Geometry check sheet. Reference: the model listing, model coordinates, mm. A direction names the side the tool comes from. Round coordinates to 2 decimals unless told otherwise and drop trailing zeros. Write each loop counter-clockwise with the first axis right and the second up, starting at its lowest first coordinate (ties: lowest second). Pieces come first, ordered by that corner, then holes. Notation, with made-up numbers: (63.5, 21) - (109.5, 21) arc R15 cw to (109.5, 35) - close; hole circle Ø4 at (26.25, -27). An arc over 180 degrees is marked (long way). Return JSON: item names as keys, results as strings.
Autodesk Inventor part; units mm, degrees
ref_plane "Work Plane4" through (-20, 152.4, 0) normal (-1, 0, 0) x (0, -1, 0)
ref_plane "YZ Plane" through (0, 0, 0) normal (1, 0, 0) x (0, 1, 0)
ref_plane "XZ Plane" through (0, 0, 0) normal (0, 1, 0) x (-1, 0, 0)
sketch "Sketch1" plane through (0, 0, 0) normal (0, 1, 0) x (-1, 0, 0)
  circle A0 centre (0, 0) radius 20
  circle A1 centre (0, 0) radius 18.5
  dimension "d0" = 40
  dimension "d1" = 1.5
extrude "Extrusion1" add sketch "Sketch1" along normal blind 152.4
sketch "Sketch4" plane through (0, 152.4, 0) normal (0, 1, 0) x (1, 0, 0)
  circle A0 centre (0, 0) radius 18.5
  circle A1 centre (0, 0) radius 20
  point P0 (-20, 0)
ref_plane "Work Plane4" through (-20, 152.4, 0) normal (-1, 0, 0) x (0, -1, 0)
sketch "Sketch8" plane through (-20, 152.4, 0) normal (-1, 0, 0) x (0, -1, 0)
  line L0 (0, 0) -> (0, 304.8) construction
  arc A0 (-304.8, 304.8) -> (0, 0) centre (0, 304.8) ccw
  line L1 (0, 304.8) -> (-304.8, 304.8) construction
  point P0 (152.4, 0)
  dimension "d7" = 304.8
sweep "Sweep1" add profiles "Sketch4" path "Sketch8"
sketch "Sketch9" plane through (0, 457.2, 304.8) normal (0, 0, 1) x (1, 0, 0)
  circle A0 centre (0, 0) radius 18.5
  circle A1 centre (0, 0) radius 20
  point P0 (0, -457.2)
extrude "Extrusion2" add sketch "Sketch9" along normal blind 152.4
properties part number "sweep" material "ABS Plastic"
(1) Release check for a two-part mould opening along Y. For faces 1 (the face through (-6, 0, -18)), 2 (the face through (18, 451, 457.2)), 3 (the face through (8.54, 473.61, 379.93)) record: pulls with the +Y half, pulls with the -Y half, needs draft (parallel to the pull), parting line crosses it, or undercut.
Response values:
{"face 1": "pulls with the -Y half", "face 2": "needs draft", "face 3": "undercut"}
(2) Access from +Z, -Z, +X, -X, +Y, -Y to the whole of each face (thin tool, end or side, straight path). Record for faces 4 (the face through (4.01, 75.13, 18.06)), 5 (the face through (10.752, 440.336, 379.933)).
Response values:
{"face 4": "-Y", "face 5": "+Z"}
(3) Material ranges on line 1 along X through (y, z) = (196, 2.5); line 2 along Z through (x, y) = (0, 98.5); line 3 along Y through (x, z) = (15, 435.5), recorded low to high. Write a range as [from, to].
Response values:
{"line 1": "x = [-19.99, -18.49], [18.49, 19.99]", "line 2": "z = [-20, -18.5], [18.5, 20]", "line 3": "y = [443.97, 446.37], [468.03, 470.43]"}
(4) Section check B-B, the plane z = 401.5. Enter the section's corners in (x, y), plus the area to 3 significant figures.
Response values:
{"outline": "circle Ø40 at (0, 457.2); hole circle Ø37 at (0, 457.2)", "area": "181 mm^2"}
(5) Gauge pin test, flat ends, axial feed: pin 1 (12 mm diameter, centred on y = 406.5, z = 99, fed in from -X); pin 2 (1 mm diameter, centred on x = 0, z = 344.5, fed in from +Y); pin 3 (8 mm diameter, centred on x = 14, y = 167, fed in from +Z). Record the tip position at first contact, or that the pin passes through.
Response values:
{"pin 1": "stops at x = -11.75", "pin 2": "stops at y = 477.2", "pin 3": "stops at z = 17.7"}
(6) Section check A-A, the plane x = 0. Enter the section's corners in (y, z), plus the area to 3 significant figures.
Response values:
{"outline": "(0, -20) - (152.4, -20) arc R324.8 ccw to (477.2, 304.8) - (477.2, 457.2) - (475.7, 457.2) - (475.7, 304.8) arc R323.3 cw to (152.4, -18.5) - (0, -18.5) - close; (0, 18.5) - (152.4, 18.5) arc R286.3 ccw to (438.7, 304.8) - (438.7, 457.2) - (437.2, 457.2) - (437.2, 304.8) arc R284.8 cw to (152.4, 20) - (0, 20) - close", "area": "2,350 mm^2"}
